from build123d import *

# Parameters (mm, degrees)
SKETCH_AS_DRAWN_R              = 25
SKETCH_AS_DRAWN_R_2            = 3
SKETCH_AS_DRAWN_R_3            = 2
EXTRUDE_DEPTH                  = 3
EXTRUDE_ONTO_SKETCH_ROLL_ANGLE = 90


with BuildPart() as part:
    # Sketch as drawn → Extrude (new)
    with BuildSketch(Plane.XY):
        Circle(SKETCH_AS_DRAWN_R)
        Circle(SKETCH_AS_DRAWN_R_2, mode=Mode.SUBTRACT)
        with Locations((0, 17)):
            Circle(SKETCH_AS_DRAWN_R_3, mode=Mode.SUBTRACT)
        with Locations((0, -17)):
            Circle(SKETCH_AS_DRAWN_R_3, mode=Mode.SUBTRACT)
    extrude(amount=-EXTRUDE_DEPTH)


with BuildPart() as part_1:
    # Extrude onto Sketch roll: moved
    add(part.part.rotate(Axis((0, 0, 0), (1, 0, 0)), EXTRUDE_ONTO_SKETCH_ROLL_ANGLE))


with BuildPart() as part_2:
    # Extrude onto Sketch placement: moved
    add(part_1.part)


with BuildPart() as part_3:
    # Extrude placement: moved
    add(part_2.part.moved(Location((0, -11, 0))))


solid = part_3.part
Verification items for the finished model (mm, model axes). Give positions to 0.01 mm unless a question says otherwise; leave off trailing zeros. Loops run counter-clockwise (first coordinate to the right, second up) from the corner with the lowest first, then second, coordinate; pieces in that order, holes last.
1. Material ranges on probe 1 along Z at (x, y) = (0, -10.1); probe 2 along Z at (x, y) = (0.5, -9.15) (1 decimal); probe 3 along X at (y, z) = (-8.6, -18.5), recorded low to high.
Derived:
probe 1: z = -25 to -19, -15 to -3, 3 to 15, 19 to 25
probe 2: z = -25 to -18.9, -15.1 to -3, 3 to 15.1, 18.9 to 25
probe 3: x = -16.82 to -1.32, 1.32 to 16.82
2. Cross-section at A-A on x = 0. Record the cut outline in (y, z).
Derived:
outline: (-11, -25) - (-8, -25) - (-8, -19) - (-11, -19) - close; (-11, -15) - (-8, -15) - (-8, -3) - (-11, -3) - close; (-11, 3) - (-8, 3) - (-8, 15) - (-11, 15) - close; (-11, 19) - (-8, 19) - (-8, 25) - (-11, 25) - close
3. Cross-section at C-C on y = -10.4. Record the cut outline in (x, z), and give its area (3 significant figures).
Derived:
outline: circle Ø50 at (0, 0); hole circle Ø6 at (0, 0); hole circle Ø4 at (0, -17); hole circle Ø4 at (0, 17)
area: 1,910 mm2
4. Release check for a two-part mould opening along X. For faces 1 (the flat face through (0, -11, -5)), 2 (the cylindrical face through (23.846, -9.521, 7.509)), 3 (the cylindrical face through (-3, -10, 0)) record: +X half, -X half, draft (parallel to the pull), parting line (faces both ways), or undercut.
Derived:
face 1: draft
face 2: parting line
face 3: undercut
5. Cross-section at B-B on z = 0. Record the cut outline in (x, y), and give its area (3 significant figures).
Derived:
outline: (-25, -11) - (-3, -11) - (-3, -8) - (-25, -8) - close; (3, -11) - (25, -11) - (25, -8) - (3, -8) - close
area: 132 mm2
6. Cross-section at D-D on z = -18. Record the cut outline in (x, y), and give its area (3 significant figures).
Derived:
outline: (-17.35, -11) - (-1.73, -11) - (-1.73, -8) - (-17.35, -8) - close; (1.73, -11) - (17.35, -11) - (17.35, -8) - (1.73, -8) - close
area: 93.7 mm2
